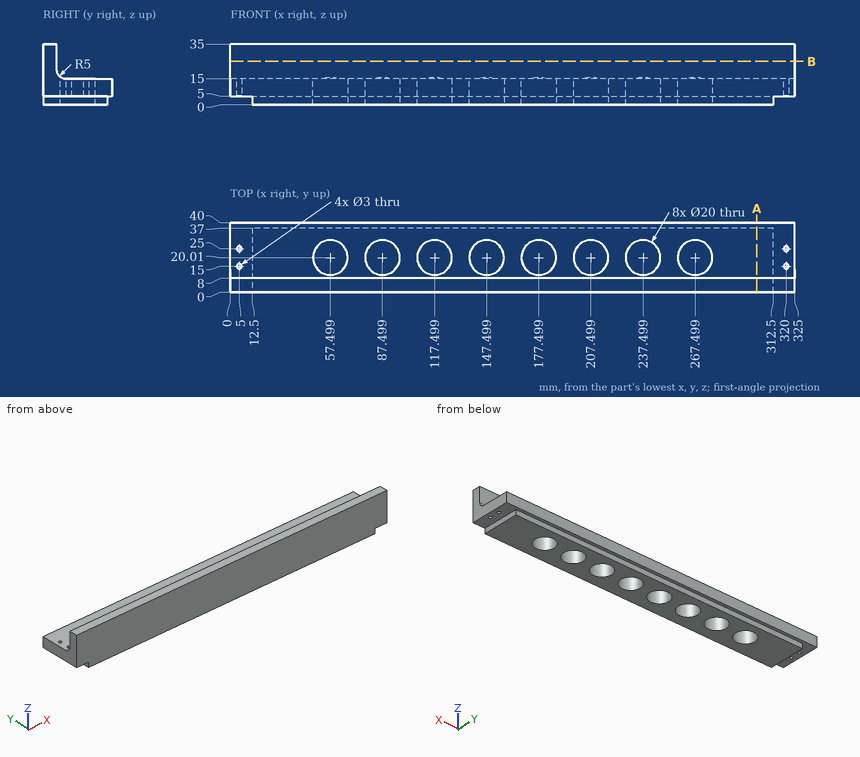
Drawing for the job (mm, zero at the part's lowest x, y, z). Round coordinates to 2 decimals unless told otherwise and drop trailing zeros. Write each loop counter-clockwise with the first axis right and the second up, starting at its lowest first coordinate (ties: lowest second). Pieces come first, ordered by that corner, then holes. Notation, with made-up numbers: M 8,0 L 31,0 A17 ccw 31,16 Z; hole C -26.5,53.5 d3. An arc over 180 degrees is marked long. Answer as a JSON object with one key per item and string values. Group by question number.
(1) Flat gauge pins, fed straight in: pin 1 (16.5 mm diameter, centred on x = 94.5, z = 29.5, fed in from +Y); pin 2 (4 mm diameter, centred on x = 320, y = 25, fed in from -Z); pin 3 (12 mm diameter, centred on x = 276.5, y = 18.5, fed in from +Z) (3 decimals). Where does each tip first touch, or does it go through?
(2) Cut at A-A (x = 303). Give the cut face in (y, z).
(3) Cut at B-B (z = 25). Give the cut face in (x, y), and give its area (3 significant figures).
(4) Drill centre lines: L1, parallel to Y at x = 207, z = 4; L2, parallel to Y at x = 5, z = 12; L3, parallel to Y at x = 189, z = 26. Where is each one in solid material? Low to high.
Responses:
{
 "1": {"pin 1": "stops at y = 8", "pin 2": "stops at z = 5", "pin 3": "stops at z = 15.025"},
 "2": {"outline": "M 0,0 L 37,0 L 37,5 L 40,5 L 40,15 L 13,15 A5 cw 8,20 L 8,35 L 0,35 Z"},
 "3": {"outline": "M 0,0 L 325,0 L 325,8 L 0,8 Z", "area": "2,600 mm2"},
 "4": {"L1": "y = 0 to 10.02, 30 to 37", "L2": "y = 0 to 13.5, 16.5 to 23.5, 26.5 to 40", "L3": "y = 0 to 8"}
}
